Study the drawing (mm; zero at the part's minimum x, y, z) and answer. A direction names the side the tool comes from. Coordinates: 2 decimals unless noted, no trailing zeros. Write each loop counter-clockwise with the first axis right and the second up, starting at its lowest first coordinate (ties: lowest second). Pieces come first, ordered by that corner, then holes. Notation, with made-up numbers: (13, 12.5) -> (54, 12.5) arc R25 ccw to (54, 45.5) -> close; hole circle Ø8 at (71.5, -2.75). An arc over 180 degrees is marked (long way). Write item = value, one per line. Start each with the question number.
1) Find the intervals of material crossed by line 1 along X through (y, z) = (32, 73); line 2 along X through (y, z) = (20, 37); line 3 along Y through (x, z) = (75, 75.5), in increasing order. Write a range as from..to.
2) For a pull along Z with two mould halves and no side action, classify the marked faces 1, 2 and 3 as released by +Z, released by -Z, zero draft, split by the parting line, or undercut.
3) Section C-C (x = 75) is taken. Count the separate pieces of the cut face and the enclosed holes in it, plus the area to 3 significant figures.
4) Flat-ended cylindrical pins translate along their axes: pin 1 Ø11 at (x, y) = (60.5, 31) entering from -Z; pin 2 Ø2 at (x, y) = (46.5, 20.5) entering from -Z; pin 3 Ø15 at (x, y) = (48, 12) entering from +Z. Find the tip coordinate at first contact, or state that the pin passes through.
5) Section B-B (z = 14) is taken. Determine the outline of the cut face in (x, y) (1 decimal).
6) A tool of negligible diameter and unlimited length cuts with its end or side. For the marked faces 4 and 5, from which of +Z, -Z, +X, -X, +Y, -Y can it reach the whole face along a straight path? Write none if from no direction.
7) Section D-D (y = 32.25) is taken. Determine the outline of the cut face in (x, z), plus the area to 4 significant figures.
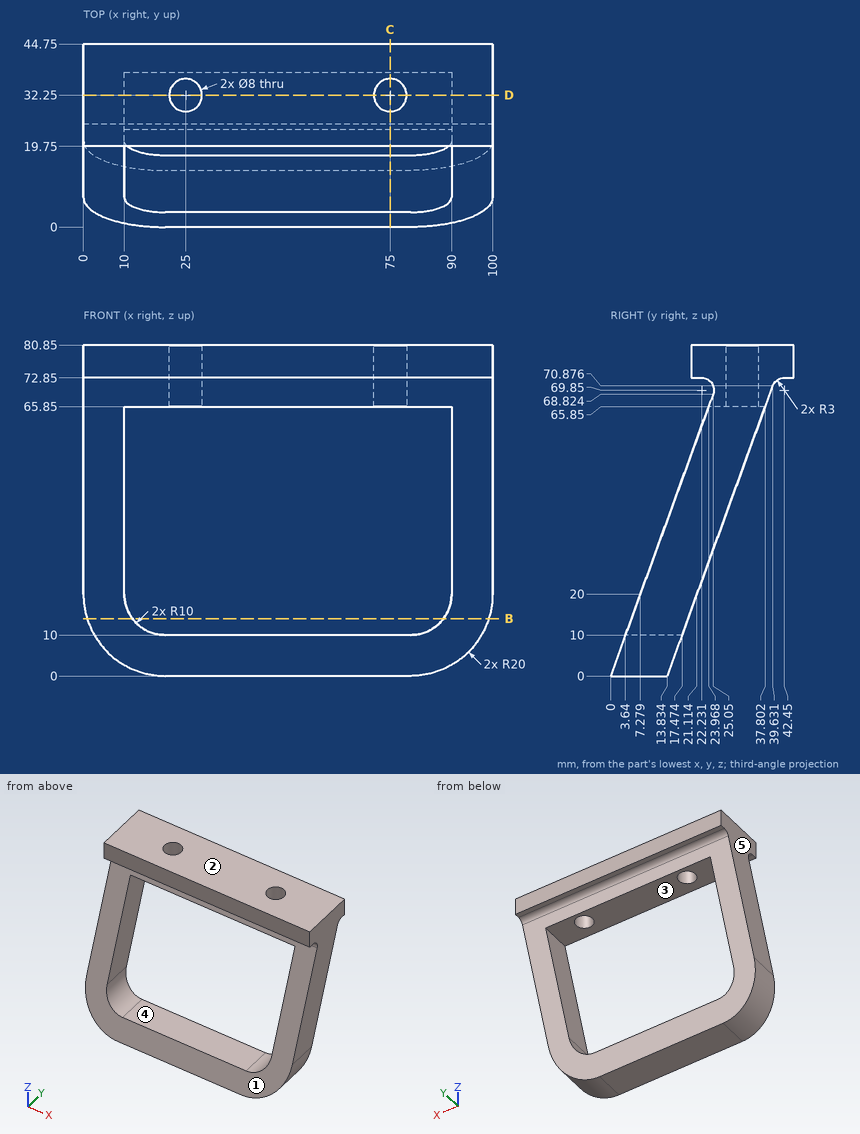
Answer key:
q1.line_1 = 0..21.01, 28.99..71.01, 78.99..100
q1.line_2 = 0..10, 90..100
q1.line_3 = 19.75..28.25, 36.25..44.75
q2.face_1 = undercut
q2.face_2 = released by +Z
q2.face_3 = released by -Z
q3.separate_pieces = 3
q3.enclosed_holes = 0
q3.area = 320 mm^2
q4.pin_1 = 65.85
q4.pin_2 = 72.85
q4.pin_3 = 10
q5.outline = (0.9, 5.1) -> (12, 5.1) -> (12, 18.9) -> (0.9, 18.9) -> close; (88, 5.1) -> (99.1, 5.1) -> (99.1, 18.9) -> (88, 18.9) -> close
q6.face_4 = +Z, +Y, -Y
q6.face_5 = +Z, -Z, -X, +Y, -Y
q7.outline = (0, 50.6) -> (10, 50.6) -> (10, 65.85) -> (21, 65.85) -> (21, 80.85) -> (0, 80.85) -> close; (29, 65.85) -> (71, 65.85) -> (71, 80.85) -> (29, 80.85) -> close; (79, 65.85) -> (90, 65.85) -> (90, 50.6) -> (100, 50.6) -> (100, 80.85) -> (79, 80.85) -> close
q7.area = 1,565 mm^2
